```python
from build123d import *

# Parameters (mm, degrees)
BOSS_EXTRUDE1_DEPTH     = 63
CUT_EXTRUDE2_DEPTH      = 65.070273919
CUT_EXTRUDE2_DEPTH_BACK = 65.070273919
SKETCH2_R               = 1.75
CUT_EXTRUDE3_START      = 1.2
SKETCH3_R               = 4
CUT_EXTRUDE3_DEPTH      = 63


with BuildPart() as part:
    # Sketch1 → Boss-Extrude1 (new body)
    with BuildSketch(Plane.XY):
        Polygon((-10, 6), (-10, 0), (10, 0), (10, 6), (9, 6), (9, 1.2), (6.833333333, 1.2), (6.833333333, 6), (5.833333333, 6), (5.833333333, 1.2), (3.666666667, 1.2), (3.666666667, 6), (2.666666667, 6), (2.666666667, 1.2), (0.5, 1.2), (0.5, 6), (-0.5, 6), (-0.5, 1.2), (-2.666666667, 1.2), (-2.666666667, 6), (-3.666666667, 6), (-3.666666667, 1.2), (-5.833333333, 1.2), (-5.833333333, 6), (-6.833333333, 6), (-6.833333333, 1.2), (-9, 1.2), (-9, 6), align=None)
    extrude(amount=-BOSS_EXTRUDE1_DEPTH)

    # Sketch2 → Cut-Extrude2 (cut, two sides: drawn at the far end of the back side and taken through both)
    with BuildSketch(Plane(origin=(0, 0, 0), x_dir=(1, 0, 0), z_dir=(0, 1, 0)).offset(-CUT_EXTRUDE2_DEPTH_BACK)):
        with Locations(Location((0, 56.9, 0), (0, 0, 253.398450401))):
            Circle(SKETCH2_R)
        with Locations(Location((0, 6.1, 0), (0, 0, 253.398450401))):
            Circle(SKETCH2_R)
    extrude(amount=CUT_EXTRUDE2_DEPTH + CUT_EXTRUDE2_DEPTH_BACK, mode=Mode.SUBTRACT)

    # Sketch3 → Cut-Extrude3 (cut)
    with BuildSketch(Plane(origin=(0, 0, 0), x_dir=(1, 0, 0), z_dir=(0, 1, 0)).offset(CUT_EXTRUDE3_START)):
        with Locations((0, 56.9)):
            Circle(SKETCH3_R)
        with Locations((0, 6.1)):
            Circle(SKETCH3_R)
    extrude(amount=CUT_EXTRUDE3_DEPTH, mode=Mode.SUBTRACT)


solid = part.part
```
For this review, take the finished solid that the model builds, in its own axes (mm). A direction names the side the tool comes from. Round coordinates to 2 decimals unless told otherwise and drop trailing zeros. Write each loop counter-clockwise with the first axis right and the second up, starting at its lowest first coordinate (ties: lowest second). Pieces come first, ordered by that corner, then holes. Notation, with made-up numbers: (-24, 24.25) -> (-20, 24.25) arc R4 ccw to (-20, 29.25) -> close; hole circle Ø6 at (31.25, -31.75). An arc over 180 degrees is marked (long way). One line per question, with ' | ' between items. Start each with the question number.
1) Add section B-B (y = 4.05). Count the separate pieces of the cut face and the enclosed holes in it, and give its area (3 significant figures).
2) Add section A-A (z = -6.1). Write out the cut boundary in (x, y), and give its area (3 significant figures).
3) Wall thickness on line 1 along X through (y, z) = (2.8, -57.5); line 2 along Z through (x, y) = (0, 0.6); line 3 along X through (y, z) = (0.5, -56.9): over which ranges is each line inside the solid? List them lowest first.
4) Mouldability with a two-part tool opening along X and no side actions: class faces 1 (the flat face through (0, 0, -31)), 2 (the flat face through (3.667, 4, -31)), 3 (the flat face through (10, 3, -31)) as +X half, -X half, draft (parallel to the pull), parting line (faces both ways), or undercut.
5) Add section C-C (z = -52). Write out the cut boundary in (x, y).
6) For pin 1 Ø4.5 at (x, z) = (0, -6.1) entering from +Y; pin 2 Ø3 at (x, z) = (0, -56.9) entering from -Y, all flat-tipped, find the tip position at first contact; note any pin that passes through.
7) Machinability: for faces 4 (the cylindrical face through (-0.624, 0.592, -7.735)), 5 (the flat face through (0.5, 4, -31)), 6 (the cylindrical face through (3.2, 3.6, -54.5)), which of the approach directions +Z, -Z, +X, -X, +Y, -Y give a long, thin tool a straight path to every point of the face, cutting with its end or side? Answer none if there is none.
Reported:
1) separate pieces: 13 | enclosed holes: 0 | area: 406 mm²
2) outline: (-10, 0) -> (-1.75, 0) -> (-1.75, 1.2) -> (-5.83, 1.2) -> (-5.83, 6) -> (-6.83, 6) -> (-6.83, 1.2) -> (-9, 1.2) -> (-9, 6) -> (-10, 6) -> close; (1.75, 0) -> (10, 0) -> (10, 6) -> (9, 6) -> (9, 1.2) -> (6.83, 1.2) -> (6.83, 6) -> (5.83, 6) -> (5.83, 1.2) -> (1.75, 1.2) -> close | area: 39.0 mm²
3) line 1: x = -10 to -9, -6.83 to -5.83, 5.83 to 6.83, 9 to 10 | line 2: z = -63 to -58.65, -55.15 to -7.85, -4.35 to 0 | line 3: x = -10 to -1.75, 1.75 to 10
4) face 1: draft | face 2: undercut | face 3: +X half
5) outline: (-10, 0) -> (10, 0) -> (10, 6) -> (9, 6) -> (9, 1.2) -> (6.83, 1.2) -> (6.83, 6) -> (5.83, 6) -> (5.83, 1.2) -> (3.67, 1.2) -> (3.67, 6) -> (2.67, 6) -> (2.67, 1.2) -> (0.5, 1.2) -> (0.5, 6) -> (-0.5, 6) -> (-0.5, 1.2) -> (-2.67, 1.2) -> (-2.67, 6) -> (-3.67, 6) -> (-3.67, 1.2) -> (-5.83, 1.2) -> (-5.83, 6) -> (-6.83, 6) -> (-6.83, 1.2) -> (-9, 1.2) -> (-9, 6) -> (-10, 6) -> close
6) pin 1: stops at y = 1.2 | pin 2: passes through
7) face 4: +Y, -Y | face 5: +Z, -Z, +Y | face 6: +Y
